Part print with two shaded views. Sizes in mm from the minimum x, y, z corner. A direction names the side the tool comes from. Coordinates: 2 decimals unless noted, no trailing zeros. Write each loop counter-clockwise with the first axis right and the second up, starting at its lowest first coordinate (ties: lowest second). Pieces come first, ordered by that corner, then holes. Notation, with made-up numbers: M -39,27 L 9,27 A17 ccw 9,34 Z; hole C -29.75,-27.75 d4. An arc over 180 degrees is marked long. One line per question, with ' | ' between items. Start each with the question number.
(1) Cut at C-C (y = 12.5). Write the cut outline in (x, z), plus the area to 3 significant figures.
(2) Tool access for the marked faces 4, 5 and 6: list every direction of +Z, -Z, +X, -X, +Y, -Y with a clear straight run to the whole face (end or side of a thin tool).
(3) Flat gauge pin, fed straight in: pin 1 Ø1.5 at (y, z) = (12.5, 6.5) entering from -X. Where does the tip first touch, or does it go through?
(4) Cut at B-B (z = 12). Write the cut outline in (x, y), plus the area to 3 significant figures.
(5) Wall check: probe 1 along X at (y, z) = (3.75, 8.5); probe 2 along Y at (x, z) = (13, 11.25); probe 3 along X at (y, z) = (2.75, 3). Give the ranges that are in metal, low to high.
(6) Cut at A-A (x = 13). Write the cut outline in (y, z), plus the area to 4 significant figures.
(7) Two-plate mould, pull along X, no slides. Class the marked faces 1, 2 and 3: +X half, -X half, draft (parallel to the pull), parting line (faces both ways), or undercut.
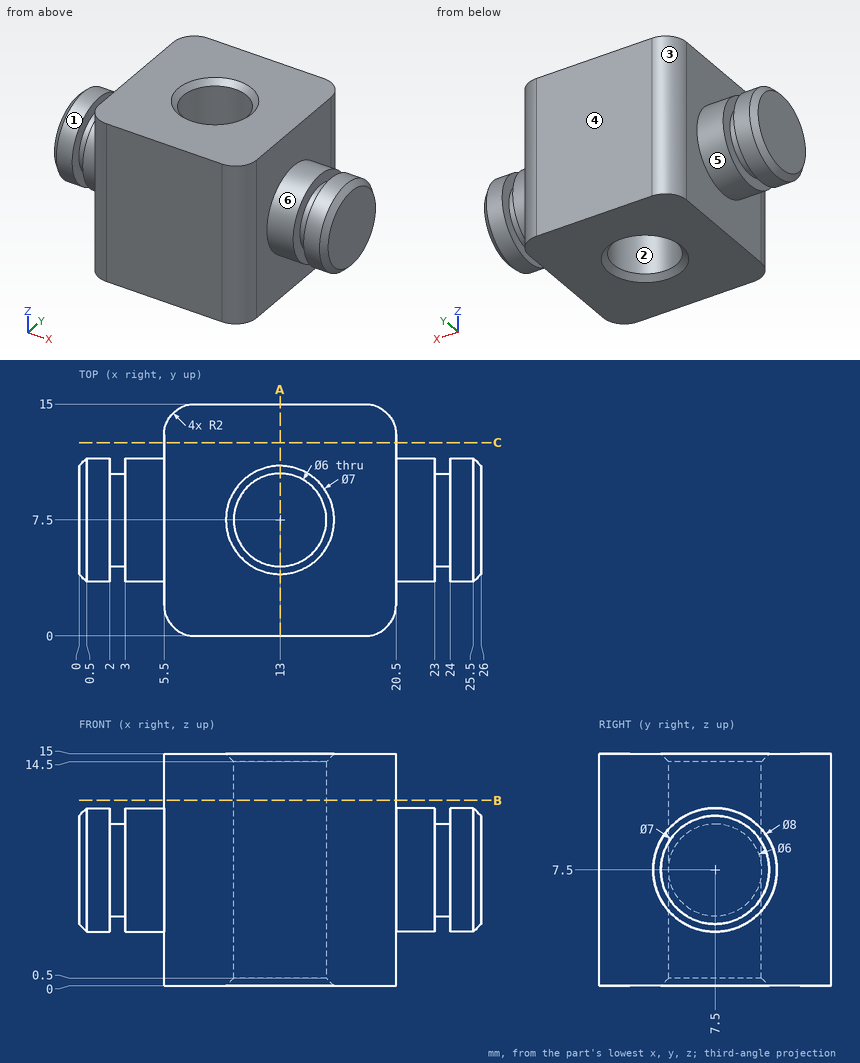
Filled in:
1) outline: M 5.5,0 L 20.5,0 L 20.5,15 L 5.5,15 Z | area: 225 mm²
2) face 4: +Z, -Z, +X, -X, +Y | face 5: -X | face 6: +X
3) pin 1: x = 5.5
4) outline: M 5.5,2 A2 ccw 7.5,0 L 18.5,0 A2 ccw 20.5,2 L 20.5,13 A2 ccw 18.5,15 L 7.5,15 A2 ccw 5.5,13 Z; hole C 13,7.5 d6 | area: 193 mm²
5) probe 1: 0.38 to 2, 3 to 23, 24 to 25.62 | probe 2: 0 to 4.5, 10.5 to 15 | probe 3: 5.5 to 20.5
6) outline: M 0,0 L 4,0 L 4.5,0.5 L 4.5,14.5 L 4,15 L 0,15 Z; M 10.5,0.5 L 11,0 L 15,0 L 15,15 L 11,15 L 10.5,14.5 Z | area: 134.5 mm²
7) face 1: draft | face 2: undercut | face 3: -X half
